```python
from build123d import *

# Parameters (mm, degrees)
BOSS_EXTRUDE1_DEPTH = 12.7
SKETCH3_W           = 78.74
SKETCH3_H           = 15.24
CUT_EXTRUDE1_DEPTH  = 15.24
SKETCH5_W           = 50.8
SKETCH5_H           = 15.24
CUT_EXTRUDE2_DEPTH  = 7.62
SKETCH6_R           = 5.08
CUT_EXTRUDE3_DEPTH  = 10.16
SKETCH7_W           = 15.24
SKETCH7_H           = 104.14
CUT_EXTRUDE4_DEPTH  = 15.24
SKETCH8_R           = 5.08
CUT_EXTRUDE5_DEPTH  = 15.24
SKETCH9_R           = 5.08
SKETCH9_R_2         = 5.375081868
SKETCH9_R_3         = 4.728276711
CUT_EXTRUDE6_DEPTH  = 15.24


with BuildPart() as part:
    # Sketch1 → Boss-Extrude1 (new body)
    with BuildSketch(Plane(origin=(0, 0, 0), x_dir=(1, 0, 0), z_dir=(0, 1, 0))):
        Polygon((0, 0), (0, 233.68), (203.2, 233.68), (203.2, 421.64), (411.48, 421.64), (411.48, 233.68), (614.68, 233.68), (614.68, 0), (411.48, 0), (411.48, -187.96), (203.2, -187.96), (203.2, 0), align=None)
    extrude(amount=BOSS_EXTRUDE1_DEPTH)

    # Sketch3 → Cut-Extrude1 (cut)
    with BuildSketch(Plane(origin=(0, 12.7, 0), x_dir=(1, 0, 0), z_dir=(0, 1, 0))):
        with Locations((242.57, 414.02)):
            Rectangle(SKETCH3_W, SKETCH3_H)
        with Locations((372.11, 414.02)):
            Rectangle(SKETCH3_W, SKETCH3_H)
        with Locations((372.11, -180.34)):
            Rectangle(SKETCH3_W, SKETCH3_H)
        with Locations((242.57, -180.34)):
            Rectangle(SKETCH3_W, SKETCH3_H)
    extrude(amount=-CUT_EXTRUDE1_DEPTH, mode=Mode.SUBTRACT)

    # Sketch5 → Cut-Extrude2 (cut)
    with BuildSketch(Plane(origin=(0, 0, 0), x_dir=(-1, 0, 0), z_dir=(0, -1, 0))):
        with Locations((-307.34, -180.34)):
            Rectangle(SKETCH5_W, SKETCH5_H)
        with Locations((-307.34, 414.02)):
            Rectangle(SKETCH5_W, SKETCH5_H)
    extrude(amount=-CUT_EXTRUDE2_DEPTH, mode=Mode.SUBTRACT)

    # Sketch6 → Cut-Extrude3 (cut)
    with BuildSketch(Plane(origin=(0, 12.7, 0), x_dir=(1, 0, 0), z_dir=(0, 1, 0))):
        with Locations(Location((307.34, 414.02, 0), (0, 0, 270))):
            Circle(SKETCH6_R)
        with Locations(Location((304.8, -180.34, 0), (0, 0, 270))):
            Circle(SKETCH6_R)
    extrude(amount=-CUT_EXTRUDE3_DEPTH, mode=Mode.SUBTRACT)

    # Sketch7 → Cut-Extrude4 (cut)
    with BuildSketch(Plane(origin=(0, 12.7, 0), x_dir=(1, 0, 0), z_dir=(0, 1, 0))):
        with Locations((7.62, 52.07)):
            Rectangle(SKETCH7_W, SKETCH7_H)
        with Locations((7.62, 181.61)):
            Rectangle(SKETCH7_W, SKETCH7_H)
        with Locations((607.06, 52.07)):
            Rectangle(SKETCH7_W, SKETCH7_H)
        with Locations((607.06, 181.61)):
            Rectangle(SKETCH7_W, SKETCH7_H)
    extrude(amount=-CUT_EXTRUDE4_DEPTH, mode=Mode.SUBTRACT)

    # Sketch8 → Cut-Extrude5 (cut)
    with BuildSketch(Plane(origin=(0, 12.7, 0), x_dir=(1, 0, 0), z_dir=(0, 1, 0))):
        with Locations(Location((607.06, 116.84, 0), (0, 0, 270))):
            Circle(SKETCH8_R)
        with Locations(Location((7.62, 116.84, 0), (0, 0, 270))):
            Circle(SKETCH8_R)
    extrude(amount=-CUT_EXTRUDE5_DEPTH, mode=Mode.SUBTRACT)

    # Sketch9 → Cut-Extrude6 (cut)
    with BuildSketch(Plane(origin=(0, 12.7, 0), x_dir=(1, 0, 0), z_dir=(0, 1, 0))):
        with Locations(Location((27.94, 226.06, 0), (0, 0, 270))):
            Circle(SKETCH9_R)
        with Locations(Location((50.8, 226.06, 0), (0, 0, 270))):
            Circle(SKETCH9_R)
        with Locations(Location((73.66, 226.06, 0), (0, 0, 270))):
            Circle(SKETCH9_R)
        with Locations(Location((96.52, 226.06, 0), (0, 0, 270))):
            Circle(SKETCH9_R)
        with Locations(Location((581.66, 226.06, 0), (0, 0, 270))):
            Circle(SKETCH9_R)
        with Locations(Location((558.8, 226.06, 0), (0, 0, 270))):
            Circle(SKETCH9_R)
        with Locations(Location((535.94, 226.06, 0), (0, 0, 270))):
            Circle(SKETCH9_R)
        with Locations(Location((513.08, 226.06, 0), (0, 0, 270))):
            Circle(SKETCH9_R)
        with Locations(Location((27.94, 7.62, 0), (0, 0, 270))):
            Circle(SKETCH9_R)
        with Locations(Location((50.8, 7.62, 0), (0, 0, 270))):
            Circle(SKETCH9_R)
        with Locations(Location((73.66, 7.62, 0), (0, 0, 270))):
            Circle(SKETCH9_R)
        with Locations(Location((96.52, 7.62, 0), (0, 0, 270))):
            Circle(SKETCH9_R)
        with Locations(Location((581.66, 7.62, 0), (0, 0, 270))):
            Circle(SKETCH9_R)
        with Locations(Location((558.8, 7.62, 0), (0, 0, 270))):
            Circle(SKETCH9_R)
        with Locations(Location((535.94, 7.62, 0), (0, 0, 270))):
            Circle(SKETCH9_R)
        with Locations(Location((513.08, 7.62, 0), (0, 0, 270))):
            Circle(SKETCH9_R)
        with Locations(Location((210.82, 393.7, 0), (0, 0, 270))):
            Circle(SKETCH9_R)
        with Locations(Location((403.86, 393.7, 0), (0, 0, 270))):
            Circle(SKETCH9_R)
        with Locations(Location((210.82, 370.84, 0), (0, 0, 270))):
            Circle(SKETCH9_R_2)
        with Locations(Location((210.82, 347.98, 0), (0, 0, 270))):
            Circle(SKETCH9_R)
        with Locations(Location((210.82, 325.12, 0), (0, 0, 270))):
            Circle(SKETCH9_R)
        with Locations(Location((403.86, 370.84, 0), (0, 0, 270))):
            Circle(SKETCH9_R)
        with Locations(Location((403.86, 347.98, 0), (0, 0, 270))):
            Circle(SKETCH9_R)
        with Locations(Location((403.86, 325.12, 0), (0, 0, 270))):
            Circle(SKETCH9_R)
        with Locations(Location((210.82, -165.1, 0), (0, 0, 270))):
            Circle(SKETCH9_R)
        with Locations(Location((403.86, -165.1, 0), (0, 0, 270))):
            Circle(SKETCH9_R)
        with Locations(Location((210.82, -142.24, 0), (0, 0, 270))):
            Circle(SKETCH9_R_3)
        with Locations(Location((210.82, -119.38, 0), (0, 0, 270))):
            Circle(SKETCH9_R)
        with Locations(Location((210.82, -96.52, 0), (0, 0, 270))):
            Circle(SKETCH9_R)
        with Locations(Location((403.86, -142.24, 0), (0, 0, 270))):
            Circle(SKETCH9_R)
        with Locations(Location((403.86, -119.38, 0), (0, 0, 270))):
            Circle(SKETCH9_R)
        with Locations(Location((403.86, -96.52, 0), (0, 0, 270))):
            Circle(SKETCH9_R)
    extrude(amount=-CUT_EXTRUDE6_DEPTH, mode=Mode.SUBTRACT)


solid = part.part
```
Geometry check sheet. Reference: the model listing, model coordinates, mm. A direction names the side the tool comes from. Coordinates: 2 decimals unless noted, no trailing zeros. Loops run counter-clockwise (first coordinate to the right, second up) from the corner with the lowest first, then second, coordinate; pieces in that order, holes last.
Item 1: Sectioned sample at B-B, the plane y = 5.25. Count the separate pieces of the cut face and the enclosed holes in it, then the cut area to 3 significant figures.
Item 2: Access from +Z, -Z, +X, -X, +Y, -Y to the whole of each face (thin tool, end or side, straight path). Record for faces 1 (the face through (302, 7.62, -414)), 2 (the face through (312, 12.7, -121)), 3 (the face through (308, 7.62, 185)).
Item 3: Thickness scan on line 1 (Z direction, x = 513.08, y = 3); line 2 (X direction, y = 6, z = 161.5); line 3 (Z direction, x = 585, y = 9.25). Record the ranges inside material, lowest first.
Item 4: Go/stop test with flat-tipped pins: pin 1 Ø6 at (x, y) = (264.5, 9) entering from -Z; pin 2 Ø6.5 at (y, z) = (9.5, -31.5) entering from -X; pin 3 Ø8 at (x, z) = (210.82, 96.52) entering from -Y; pin 4 Ø6 at (y, z) = (3.5, -305) entering from +X. Record where each tip stops, or that it passes through.
Item 5: Sectioned sample at A-A, the plane x = 476. Record the boundary of the cut face in (y, z).
Item 6: Sectioned sample at C-C, the plane z = -140. Record the boundary of the cut face in (x, y), then the cut area to 3 significant figures.
Check result:
1. separate pieces: 1
1. enclosed holes: 34
1. area: 206,000 mm2
2. face 1: -Z, +X, -X, -Y
2. face 2: +Z, -Z, +X, -X, +Y
2. face 3: +Z, +X, -X, -Y
3. line 1: z = -233.68 to -231.14, -220.98 to -12.7, -2.54 to 0
3. line 2: x = 203.2 to 207.24, 214.4 to 400.28, 407.44 to 411.48
3. line 3: z = -233.68 to -229.89, -222.23 to -11.45, -3.79 to 0
4. pin 1: stops at z = -406.4
4. pin 2: stops at x = 15.24
4. pin 3: passes through
4. pin 4: stops at x = 411.48
5. outline: (0, -233.68) - (12.7, -233.68) - (12.7, 0) - (0, 0) - close
6. outline: (15.24, 0) - (599.44, 0) - (599.44, 12.7) - (15.24, 12.7) - close
6. area: 7,420 mm2
